```python
from build123d import *

# Parameters (mm, degrees)
SKETCH_W        = 50
SKETCH_H        = 30
PAD_DEPTH       = 8.25
SKETCH001_R     = 2.3
POCKET_DEPTH    = 8.251
SKETCH002_R     = 2.7
POCKET001_DEPTH = 8.251
SKETCH003_R     = 5.5
POCKET002_DEPTH = 4.75
FILLET_R        = 3
FILLET001_R     = 1


with BuildPart() as part:
    # Sketch → Pad (new body)
    with BuildSketch(Plane.XY):
        with Locations((25, 15)):
            Rectangle(SKETCH_W, SKETCH_H)
    extrude(amount=PAD_DEPTH)

    # Sketch001 (on Face6 of Pad) → Pocket (cut, through all)
    with BuildSketch(Plane.XY.offset(8.25)):
        with Locations((27.5, 23)):
            Circle(SKETCH001_R)
        with Locations((27.5, 7)):
            Circle(SKETCH001_R)
        with Locations((11.5, 7)):
            Circle(SKETCH001_R)
    extrude(amount=-POCKET_DEPTH, mode=Mode.SUBTRACT)

    # Sketch002 (on Face5 of Pocket) → Pocket001 (cut, through all)
    with BuildSketch(Plane.XY.offset(8.25)):
        with Locations((17.5, 15)):
            Circle(SKETCH002_R)
        with Locations((43.75, 15)):
            Circle(SKETCH002_R)
    extrude(amount=-POCKET001_DEPTH, mode=Mode.SUBTRACT)

    # Sketch003 (on Face5 of Pocket001) → Pocket002 (cut)
    with BuildSketch(Plane.XY.offset(8.25)):
        with Locations((43.75, 15)):
            Circle(SKETCH003_R)
        with Locations((17.5, 15)):
            Circle(SKETCH003_R)
    extrude(amount=-POCKET002_DEPTH, mode=Mode.SUBTRACT)

    # Fillet
    fillet_edges = [part.edges().sort_by_distance(p)[0] for p in [
        (50, 0, 4.125),
        (50, 30, 4.125),
        (0, 30, 4.125),
        (0, 0, 4.125),
    ]]
    fillet(fillet_edges, radius=FILLET_R)

    # Fillet001
    fillet001_edges = [part.edges().sort_by_distance(p)[0] for p in [
        (0, 15, 8.25),
        (0.87868, 29.12132, 8.25),
        (25, 30, 8.25),
        (49.12132, 29.12132, 8.25),
        (50, 15, 8.25),
        (49.12132, 0.87868, 8.25),
        (25, 0, 8.25),
        (0.87868, 0.87868, 8.25),
    ]]
    fillet(fillet001_edges, radius=FILLET001_R)


solid = part.part
```
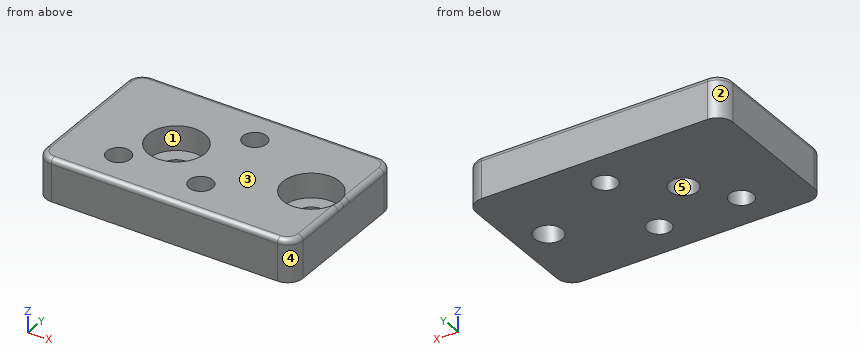
Verification items for the finished model (mm, model axes). Face numbers are marked on the shaded views. A direction names the side the tool comes from. Round coordinates to 2 decimals unless told otherwise and drop trailing zeros. Write each loop counter-clockwise with the first axis right and the second up, starting at its lowest first coordinate (ties: lowest second). Pieces come first, ordered by that corner, then holes.
1. Draft check along Y on the marked faces 3, 4 and 5. Enter one of: +Y half, -Y half, draft (parallel to the pull), parting line (faces both ways), or undercut.
2. Section check C-C on x = 11.5. Enter the section's corners in (y, z), plus the area to 3 significant figures.
3. Gauge pin test, flat ends, axial feed: P1, Ø3, axis at x = 43.75, y = 15, coming from the +Z side; P2, Ø6, axis at x = 17.5, y = 15, coming from the +Z side. Record the tip position at first contact, or that the pin passes through.
4. Scan lines: L1, parallel to Y at x = 27.5, z = 2.25; L2, parallel to Y at x = 17.5, z = 1.8; L3, parallel to X at y = 6.75, z = 1. Record each from-to range of solid material in increasing order.
5. Section check B-B on y = 7. Enter the section's corners in (x, z).
6. Section check A-A on z = 6. Enter the section's corners in (x, y).
7. Section check D-D on x = 27.5. Enter the section's corners in (y, z).
8. Access from +Z, -Z, +X, -X, +Y, -Y to the whole of each face (thin tool, end or side, straight path). Record for the marked faces 1 and 2.
Answer:
1. face 3: draft
1. face 4: -Y half
1. face 5: undercut
2. outline: (0, 0) - (4.7, 0) - (4.7, 8.25) - (1, 8.25) arc R1 ccw to (0, 7.25) - close; (9.3, 0) - (30, 0) - (30, 7.25) arc R1 ccw to (29, 8.25) - (9.3, 8.25) - close
2. area: 209 mm2
3. P1: passes through
3. P2: stops at z = 3.5
4. L1: y = 0 to 4.7, 9.3 to 20.7, 25.3 to 30
4. L2: y = 0 to 12.3, 17.7 to 30
4. L3: x = 0 to 9.21, 13.79 to 25.21, 29.79 to 50
5. outline: (0, 0) - (9.2, 0) - (9.2, 8.25) - (1, 8.25) arc R1 ccw to (0, 7.25) - close; (13.8, 0) - (25.2, 0) - (25.2, 8.25) - (13.8, 8.25) - close; (29.8, 0) - (50, 0) - (50, 7.25) arc R1 ccw to (49, 8.25) - (29.8, 8.25) - close
6. outline: (0, 3) arc R3 ccw to (3, 0) - (47, 0) arc R3 ccw to (50, 3) - (50, 27) arc R3 ccw to (47, 30) - (3, 30) arc R3 ccw to (0, 27) - close; hole circle Ø4.6 at (11.5, 7); hole circle Ø11 at (17.5, 15); hole circle Ø4.6 at (27.5, 7); hole circle Ø4.6 at (27.5, 23); hole circle Ø11 at (43.75, 15)
7. outline: (0, 0) - (4.7, 0) - (4.7, 8.25) - (1, 8.25) arc R1 ccw to (0, 7.25) - close; (9.3, 0) - (20.7, 0) - (20.7, 8.25) - (9.3, 8.25) - close; (25.3, 0) - (30, 0) - (30, 7.25) arc R1 ccw to (29, 8.25) - (25.3, 8.25) - close
8. face 1: +Z
8. face 2: +Z, -Z, -X, +Y
